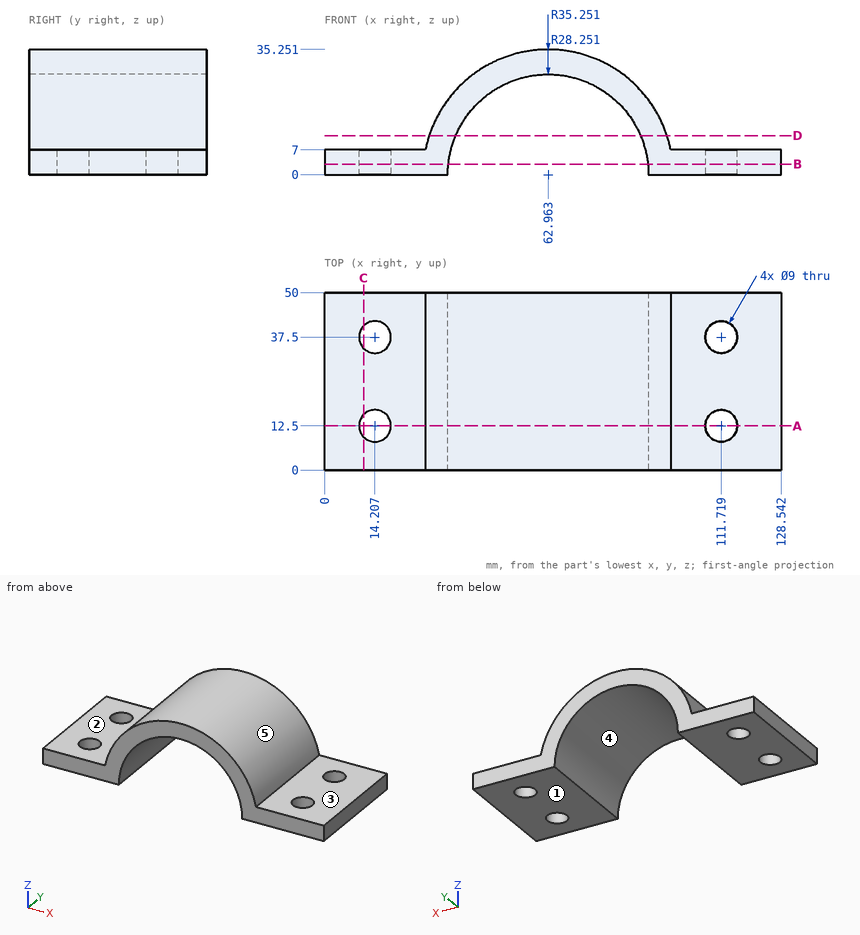
Study the drawing (mm; zero at the part's minimum x, y, z) and answer. A direction names the side the tool comes from. Round coordinates to 2 decimals unless told otherwise and drop trailing zeros. Write each loop counter-clockwise with the first axis right and the second up, starting at its lowest first coordinate (ties: lowest second). Pieces come first, ordered by that corner, then holes.
Q1. Find section D-D on z = 11. Determine the outline of the cut face in (x, y).
Values:
outline: (29.47, 0) - (36.94, 0) - (36.94, 50) - (29.47, 50) - close; (88.98, 0) - (96.45, 0) - (96.45, 50) - (88.98, 50) - close
Q2. Flat-ended cylindrical pins translate along their axes: P1, Ø5.5, axis at x = 14.21, y = 37.5, coming from the -Z side; P2, Ø1.5, axis at x = 61, y = 22, coming from the +Z side; P3, Ø4, axis at x = 79.5, y = 44.5, coming from the -Z side; P4, Ø8, axis at y = 12.5, z = 20, coming from the -X side. Find the tip coordinate at first contact, or state that the pin passes through.
Values:
P1: passes through
P2: stops at z = 35.23
P3: stops at z = 21.32
P4: stops at x = 31.55
Q3. Find section C-C on x = 11. Determine the outline of the cut face in (y, z).
Values:
outline: (0, 0) - (9.34, 0) - (9.34, 7) - (0, 7) - close; (15.66, 0) - (34.34, 0) - (34.34, 7) - (15.66, 7) - close; (40.66, 0) - (50, 0) - (50, 7) - (40.66, 7) - close
Q4. Find section B-B on z = 3. Determine the outline of the cut face in (x, y), and give its area (3 significant figures).
Values:
outline: (0, 0) - (34.87, 0) - (34.87, 50) - (0, 50) - close; (91.05, 0) - (128.54, 0) - (128.54, 50) - (91.05, 50) - close; hole circle Ø9 at (14.21, 12.5); hole circle Ø9 at (14.21, 37.5); hole circle Ø9 at (111.72, 12.5); hole circle Ø9 at (111.72, 37.5)
area: 3,360 mm2
Q5. Straight lines are drawn through the part: line 1 (X direction, y = 13.5, z = 6.5) (1 decimal); line 2 (Z direction, x = 122.5, y = 12.5); line 3 (X direction, y = 12, z = 2) (1 decimal). For each, find the intervals that lie inside material, in ascending order.
Values:
line 1: x = 0 to 9.8, 18.6 to 35.5, 90.5 to 107.3, 116.1 to 128.5
line 2: z = 0 to 7
line 3: x = 0 to 9.7, 18.7 to 34.8, 91.1 to 107.2, 116.2 to 128.5
Q6. A tool of negligible diameter and unlimited length cuts with its end or side. For the marked faces 1 and 2, from which of +Z, -Z, +X, -X, +Y, -Y can it reach the whole face along a straight path? Write none if from no direction.
Values:
face 1: -Z, +X, -X, +Y, -Y
face 2: +Z, -X, +Y, -Y
Q7. The mould has two halves that part along X. Classify the marked faces 3, 4 and 5: released by +X, released by -X, zero draft, split by the parting line, or undercut.
Values:
face 3: zero draft
face 4: undercut
face 5: split by the parting line
Q8. Find section A-A on y = 12.5. State how many separate pieces and enclosed holes the cut face has, and give its area (3 significant figures).
Values:
separate pieces: 3
enclosed holes: 0
area: 982 mm2
